Can you work these out from the model? Positions are in its coordinate system, mm. Face numbers are marked on the shaded views. A direction names the side the tool comes from. Give positions to 0.01 mm unless a question says otherwise; leave off trailing zeros. Order: outer loops, then holes, each group sorted by start corner. A loop starts at its lowest first (then second) coordinate and runs counter-clockwise, first axis right, second up. Notation, with made-up numbers: (51, 51.5) -> (79, 51.5) arc R29 cw to (79, 72.5) -> close; hole circle Ø11 at (41, 29). An arc over 180 degrees is marked (long way). Answer as a JSON object with one key per item and string values.
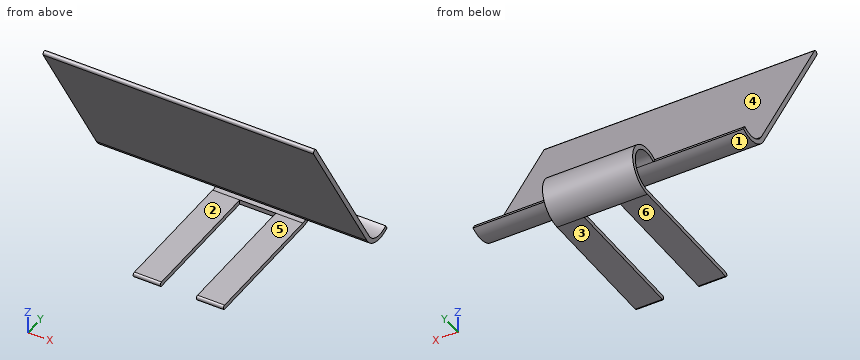
```python
from build123d import *

# Parameters (mm, degrees)
BOSS_EXTRUDE1_DEPTH      = 76.2
BOSS_EXTRUDE1_DEPTH_BACK = 76.2
BOSS_EXTRUDE3_DEPTH      = 25.4
BOSS_EXTRUDE3_DEPTH_BACK = 25.4
CUT_EXTRUDE2_DEPTH       = 3.81


with BuildPart() as part:
    # Sketch1 → Boss-Extrude1 (new, two sides: drawn at the far end of the back side and taken through both)
    with BuildSketch(Plane.YZ.offset(-BOSS_EXTRUDE1_DEPTH_BACK)):
        with BuildLine():
            Line((1.099852263, 0.635), (-49.698657582, 88.6206))
            ThreePointArc((-49.698657582, 88.6206), (-51.433509845, 89.085452263), (-51.898362108, 87.3506))
            Line((-51.898362108, 87.3506), (-1.099852263, -0.635))
            ThreePointArc((-1.099852263, -0.635), (7.382820568, -7.143983793), (17.983522628, -5.748374891))
            Line((17.983522628, -5.748374891), (16.713522628, -3.548670365))
            ThreePointArc((16.713522628, -3.548670365), (8.040220943, -4.690532194), (1.099852263, 0.635))
        make_face()
    extrude(amount=BOSS_EXTRUDE1_DEPTH + BOSS_EXTRUDE1_DEPTH_BACK)

    # Sketch1_5 → Boss-Extrude3 (add, two sides: drawn at the far end of the back side and taken through both)
    with BuildSketch(Plane.YZ.offset(-BOSS_EXTRUDE3_DEPTH_BACK)):
        with BuildLine():
            ThreePointArc((-50.798509845, -29.617045256), (-52.068509845, -28.347045256), (-50.798509845, -27.077045256))
            Line((-50.798509845, -27.077045256), (23.698522628, -27.077045256))
            ThreePointArc((23.698522628, -27.077045256), (34.739054823, -12.688743571), (17.983522628, -5.748374891))
            Line((17.983522628, -5.748374891), (16.713522628, -3.548670365))
            ThreePointArc((16.713522628, -3.548670365), (37.192506421, -12.031343196), (23.698522628, -29.617045256))
            Line((23.698522628, -29.617045256), (-50.798509845, -29.617045256))
        make_face()
    extrude(amount=BOSS_EXTRUDE3_DEPTH + BOSS_EXTRUDE3_DEPTH_BACK)

    # Sketch5 → Cut-Extrude2 (cut)
    with BuildSketch(Plane(origin=(0, 0, -29.617045256), x_dir=(1, 0, 0), z_dir=(0, 0, -1))):
        Polygon((10.16, 50.798509845), (10.16, -23.698522628), (-10.16, -23.698522628), (-10.16, 50.798509845), (-10.16, 53.498166753), (0, 53.498166753), (10.16, 53.498166753), align=None)
    extrude(amount=-CUT_EXTRUDE2_DEPTH, mode=Mode.SUBTRACT)


solid = part.part
```
1. If we mould it in two halves opening along Z, with no side actions, what happens to the marked faces 4, 5 and 6? For each: +Z half, -Z half, draft (parallel to the pull), parting line (faces both ways), or undercut.
Worked answers:
{"face 4": "+Z half", "face 5": "undercut", "face 6": "-Z half"}
2. If we section it at B-B on y = -29: Please give me the cut outline in (x, z), then the cut area to 3 significant figures.
Worked answers:
{"outline": "(-76.2, 47.69) -> (76.2, 47.69) -> (76.2, 52.77) -> (-76.2, 52.77) -> close; (-25.4, -29.62) -> (-10.16, -29.62) -> (-10.16, -27.08) -> (-25.4, -27.08) -> close; (10.16, -29.62) -> (25.4, -29.62) -> (25.4, -27.08) -> (10.16, -27.08) -> close", "area": "852 mm²"}
3. Will these pins go through, and if not, where does the flat tip stop? pin 1 Ø1.3 at (y, z) = (-5, -28) entering from +X; pin 2 Ø0.8 at (x, z) = (0, -28.5) entering from -Y; pin 3 Ø6 at (x, y) = (-34, -31) entering from -Z.
Worked answers:
{"pin 1": "x = 25.4", "pin 2": "y = 23.7", "pin 3": "z = 45.96"}
4. For the marked faces 1, 2 and 3, which set-ups out of +Z, -Z, +X, -X, +Y, -Y let a thin tool reach every point of the face, with its end or its side?
Worked answers:
{"face 1": "+X, -X", "face 2": "+X, -X, -Y", "face 3": "-Z, +X, -X, +Y, -Y"}
5. If we section it at D-D on y = 14: Please give me the cut outline in (x, z).
Worked answers:
{"outline": "(-76.2, -7.29) -> (76.2, -7.29) -> (76.2, -4.68) -> (-76.2, -4.68) -> close; (-25.4, -29.62) -> (-10.16, -29.62) -> (-10.16, -27.08) -> (-25.4, -27.08) -> close; (10.16, -29.62) -> (25.4, -29.62) -> (25.4, -27.08) -> (10.16, -27.08) -> close"}
6. Please list where these lines run through material, in increasing order: L1, parallel to Z at x = 6, y = 31.5; L2, parallel to Z at x = -2, y = 27; L3, parallel to Y at x = -1.5, z = 2.
Worked answers:
{"L1": "-27.24 to -24, -7.29 to -4.06", "L2": "-29.22 to -26.59, -4.7 to -2.07", "L3": "-2.62 to 0.31"}
